Geometry: final body of the model. Coordinates: model frame, mm. Give positions to 0.01 mm unless a question says otherwise; leave off trailing zeros. Order: outer loops, then holes, each group sorted by start corner. A loop starts at its lowest first (then second) coordinate and runs counter-clockwise, first axis right, second up. Notation, with made-up numbers: (55.5, 46.5) -> (60.5, 46.5) arc R29 cw to (60.5, 76.5) -> close; hole circle Ø8 at (85, 71). An arc over 180 degrees is marked (long way). One line per question, with ' | ' between items.
from build123d import *

# Parameters (mm, degrees)
SKETCH1_R           = 30
SKETCH1_R_2         = 24.5
BOSS_EXTRUDE1_DEPTH = 40
CHAMFER1_SIZE       = 7
CHAMFER1_SIZE2      = 2.54779164
FILLET1_R           = 1


with BuildPart() as part:
    # Sketch1 → Boss-Extrude1 (new body)
    with BuildSketch(Plane.XY):
        Circle(SKETCH1_R)
        Circle(SKETCH1_R_2, mode=Mode.SUBTRACT)
    extrude(amount=BOSS_EXTRUDE1_DEPTH)

    # Chamfer1
    chamfer1_edges = [part.edges().sort_by_distance(p)[0] for p in [
        (-30, 0, 40),
    ]]
    chamfer1_side = [part.faces().sort_by_distance(p)[0] for p in [
        (-30, 0, 20),
    ]]
    chamfer(chamfer1_edges, length=CHAMFER1_SIZE, length2=CHAMFER1_SIZE2, reference=chamfer1_side[0])

    # Fillet1
    fillet1_edges = [part.edges().sort_by_distance(p)[0] for p in [
        (-30, 0, 0),
        (-27.45220836, 0, 40),
    ]]
    fillet(fillet1_edges, radius=FILLET1_R)


solid = part.part
1) Section D-D on z = 36. Return loops of the section in (x, y), plus the area to 3 significant figures.
Check result:
outline: circle Ø57.82 at (0, 0); hole circle Ø49 at (0, 0) | area: 740 mm^2
2) Section C-C on z = 10. Return loops of the section in (x, y).
Check result:
outline: circle Ø60 at (0, 0); hole circle Ø49 at (0, 0)
3) Material intervals for probe 1 along Y at (x, z) = (0, 14); probe 2 along X at (y, z) = (-19.5, 14); probe 3 along Z at (x, y) = (23, -14), sorted ascending. Write a range as from..to.
Check result:
probe 1: y = -30..-24.5, 24.5..30 | probe 2: x = -22.8..-14.83, 14.83..22.8 | probe 3: z = 0..39.98
4) Pull-direction query (X, two-part tool) for faces 1 (the cylindrical face through (13.17, 20.66, 19.72)), 2 (the conical face through (-6.027, -27.143, 39.034)), 3 (the flat face through (-7, 24, 0)); classes: +X half, -X half, draft (parallel to the pull), parting line (faces both ways), or undercut.
Check result:
face 1: undercut | face 2: parting line | face 3: draft
5) Contact query for flat-ended pins moving along their axis: pin 1 Ø6 at (x, z) = (23.5, 28) entering from -Y; pin 2 Ø2 at (y, z) = (-3, 27.5) entering from +X; pin 3 Ø8 at (y, z) = (12.5, 29.5) entering from +X. Output: stop coordinate, or through.
Check result:
pin 1: stops at y = -21.9 | pin 2: stops at x = 29.93 | pin 3: stops at x = 28.77
6) Section A-A on x = 0. Return loops of the section in (y, z), plus the area to 3 significant figures.
Check result:
outline: (-30, 1) arc R1 ccw to (-29, 0) -> (-24.5, 0) -> (-24.5, 40) -> (-26.75, 40) arc R1 ccw to (-27.69, 39.34) -> (-30, 33) -> close; (24.5, 0) -> (29, 0) arc R1 ccw to (30, 1) -> (30, 33) -> (27.69, 39.34) arc R1 ccw to (26.75, 40) -> (24.5, 40) -> close | area: 422 mm^2
